Design review of the part shown in the three views and the two pictorial views. Dimensions are in mm from the part's minimum x, y and z. A direction names the side the tool comes from. Coordinates: 2 decimals unless noted, no trailing zeros. Loops run counter-clockwise (first coordinate to the right, second up) from the corner with the lowest first, then second, coordinate; pieces in that order, holes last. Notation, with made-up numbers: (19, -3.5) -> (57, -3.5) arc R23 cw to (57, 10.5) -> close; hole circle Ø7 at (-29.75, 10.25). An arc over 180 degrees is marked (long way). Use a Markdown table: item, result. Add a question column.
Q1. For the marked faces 1, 2 and 3, list the 3-axis set-ups (+Z, -Z, +X, -X, +Y, -Y) from which the entire face can be reached by the end or side of a thin tool; tool diameter is ignored.
Q2. Take a section at A-A on y = 152. Write out the cut boundary in (x, z).
Q3. For probe 1 along Y at (x, z) = (15, 17.75); probe 2 along X at (y, z) = (111, 22.5); probe 3 along Z at (x, y) = (14.25, 203), list the stretches that pass through material, from the lowest coordinate up.
Q4. Clearance check with flat-ended pins moving along their axes: pin 1 Ø10 at (x, y) = (9, 99.5) entering from -Z; pin 2 Ø3 at (y, z) = (184.5, 19.5) entering from +X (3 decimals); pin 3 Ø1.5 at (x, y) = (8, 186.5) entering from +Z; pin 4 Ø2 at (x, z) = (6, 17.5) entering from -Y. State where each tip first meets the part, or that it passes through.
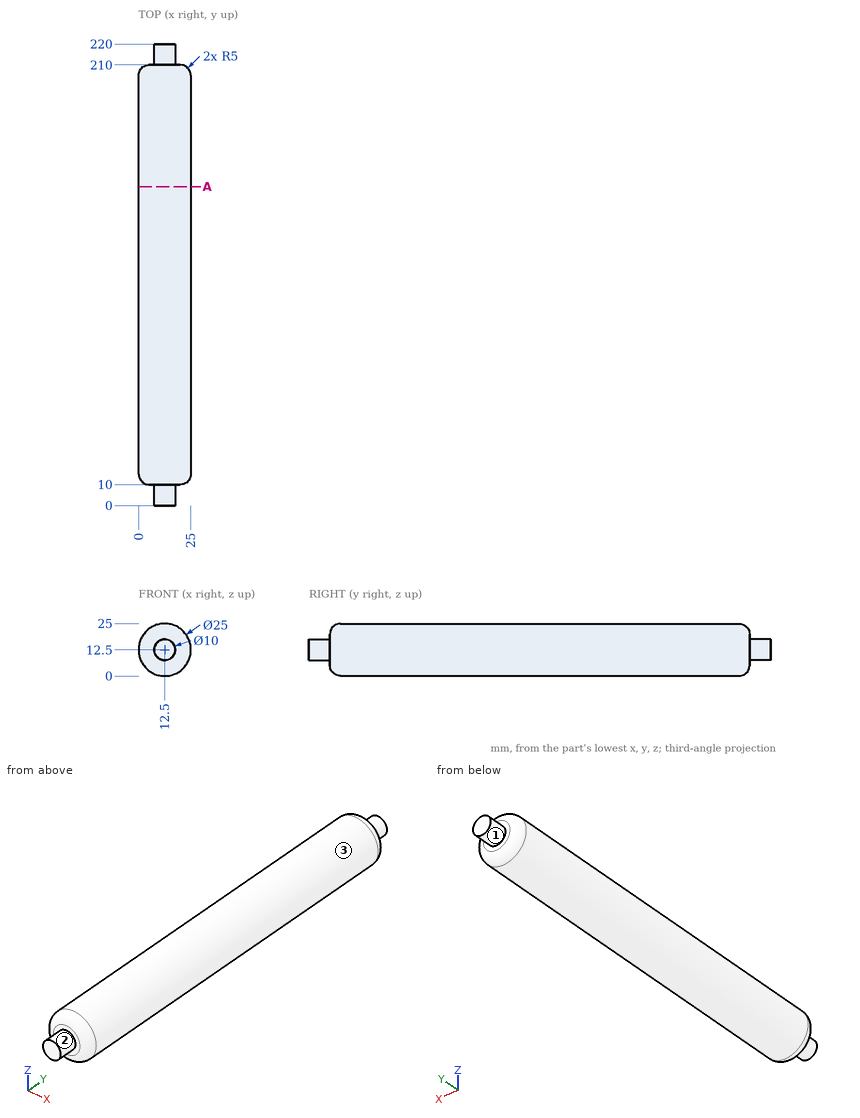
Answer list:
| question | item | result |
|---|---|---|
| 1 | face 1 | +Y |
| 1 | face 2 | -Y |
| 1 | face 3 | +Y, -Y |
| 2 | outline | circle Ø25 at (12.5, 12.5) |
| 3 | probe 1 | 10 to 210 |
| 3 | probe 2 | 5 to 20 |
| 3 | probe 3 | 0.12 to 24.88 |
| 4 | pin 1 | z = 0 |
| 4 | pin 2 | x = 23.725 |
| 4 | pin 3 | z = 24.42 |
| 4 | pin 4 | y = 10 |
